Part print with two shaded views. Sizes in mm from the minimum x, y, z corner. Give positions to 0.01 mm unless a question says otherwise; leave off trailing zeros. Write each loop counter-clockwise with the first axis right and the second up, starting at its lowest first coordinate (ties: lowest second). Pieces come first, ordered by that corner, then holes.
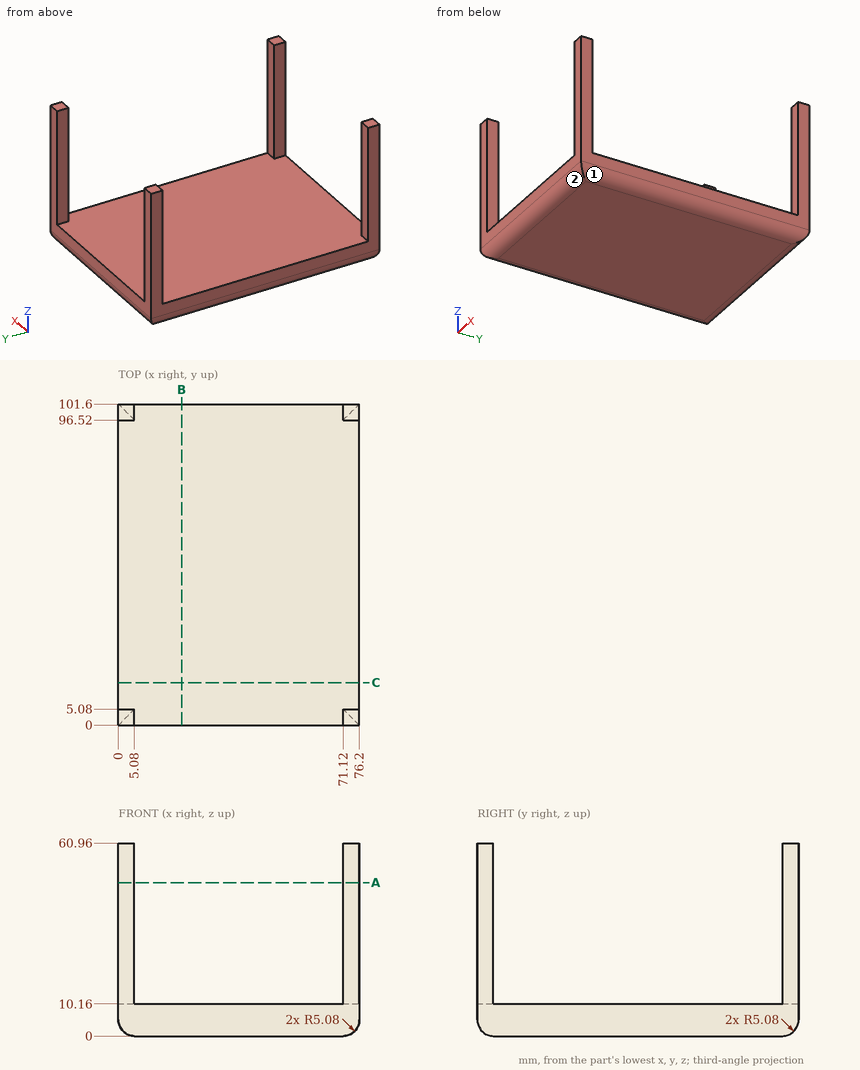
1) Saw through at B-B (x = 20). Write the cut outline in (y, z), and give its area (3 significant figures).
Check result:
outline: (0, 5.08) arc R5.08 ccw to (5.08, 0) - (96.52, 0) arc R5.08 ccw to (101.6, 5.08) - (101.6, 10.16) - (0, 10.16) - close
area: 1,020 mm2
2) Mould opens along X. For the marked faces 1 and 2 say: +X half, -X half, draft (parallel to the pull), parting line (faces both ways), or undercut.
Check result:
face 1: +X half
face 2: draft
3) Saw through at A-A (z = 48.5). Write the cut outline in (x, y).
Check result:
outline: (0, 0) - (5.08, 0) - (5.08, 5.08) - (0, 5.08) - close; (0, 96.52) - (5.08, 96.52) - (5.08, 101.6) - (0, 101.6) - close; (71.12, 0) - (76.2, 0) - (76.2, 5.08) - (71.12, 5.08) - close; (71.12, 96.52) - (76.2, 96.52) - (76.2, 101.6) - (71.12, 101.6) - close
4) Drill centre lines: L1, parallel to Y at x = 3.5, z = 16; L2, parallel to Z at x = 63.5, y = 57; L3, parallel to X at y = 9, z = 4. Where is each one in solid material? Low to high.
Check result:
L1: y = 0 to 5.08, 96.52 to 101.6
L2: z = 0 to 10.16
L3: x = 0.12 to 76.08
5) Saw through at C-C (y = 13.5). Write the cut outline in (x, z), and give its area (3 significant figures).
Check result:
outline: (0, 5.08) arc R5.08 ccw to (5.08, 0) - (71.12, 0) arc R5.08 ccw to (76.2, 5.08) - (76.2, 10.16) - (0, 10.16) - close
area: 763 mm2
6) Flat gauge pin, fed straight in: P1, Ø2, axis at x = 41.5, y = 47.5, coming from the +Z side. Where does the tip first touch, or does it go through?
Check result:
P1: stops at z = 10.16
